```python
from build123d import *

# Parameters (mm, degrees)
SALIENTE_EXTRUIR3_DEPTH = 10
CROQUIS4_W              = 20
CROQUIS4_H              = 5
SALIENTE_EXTRUIR4_DEPTH = 10
CROQUIS5_W              = 5
CROQUIS5_H              = 5
SALIENTE_EXTRUIR5_DEPTH = 20
CORTAR_EXTRUIR1_DEPTH   = 2
CROQUIS8_W              = 20
CROQUIS8_H              = 5
CORTAR_EXTRUIR2_DEPTH   = 2
CROQUIS9_W              = 5
CROQUIS9_H              = 20
CORTAR_EXTRUIR3_DEPTH   = 2
CROQUIS10_W             = 20
CROQUIS10_H             = 5
CORTAR_EXTRUIR5_DEPTH   = 35
SALIENTE_EXTRUIR6_DEPTH = 5
CROQUIS12_W             = 26.103344273
CROQUIS12_H             = 18.453448341
CORTAR_EXTRUIR6_DEPTH   = 0.25


with BuildPart() as part:
    # Croquis1 → Saliente-Extruir3 (new body)
    with BuildSketch(Plane(origin=(0, 0, 0), x_dir=(1, 0, 0), z_dir=(0, 1, 0))):
        Polygon((-12.713671106, 38.358548308), (-10.713671106, 38.358548308), (-10.713671106, 39.358548308), (-15.713671106, 39.358548308), (-15.713671106, 19.358548308), (-10.713671106, 19.358548308), (-10.713671106, 20.358548308), (-12.713671106, 20.358548308), (-12.713671106, 21.358548308), (-10.718625385, 21.358548308), (-10.718625385, 37.358548308), (-12.713671106, 37.358548308), align=None)
    extrude(amount=SALIENTE_EXTRUIR3_DEPTH)



with BuildPart() as body_2:
    # Croquis4 → Saliente-Extruir4 (new body)
    with BuildSketch(Plane(origin=(-10.713671106, 0, 0), x_dir=(0, 0, -1), z_dir=(1, 0, 0))):
        with Locations((29.358548308, -2.5)):
            Rectangle(CROQUIS4_W, CROQUIS4_H)
    extrude(amount=SALIENTE_EXTRUIR4_DEPTH)


with BuildPart() as part_1:
    add(part.part)

    add(body_2.part)  # Saliente-Extruir5 merges body 2
    # Croquis5 → Saliente-Extruir5 (add)
    with BuildSketch(Plane.XY.offset(-19.358548308)):
        with Locations((-13.213671106, -2.5)):
            Rectangle(CROQUIS5_W, CROQUIS5_H)
    extrude(amount=-SALIENTE_EXTRUIR5_DEPTH)

    # Croquis7 → Cortar-Extruir1 (cut)
    with BuildSketch(Plane(origin=(0, 0, 0), x_dir=(1, 0, 0), z_dir=(0, 1, 0))):
        Polygon((-10.714909676, 37.358548308), (-0.713671106, 37.358548308), (-0.713671106, 38.358548308), (-10.713671106, 38.358548308), (-12.713671106, 38.358548308), (-12.713671106, 37.358548308), align=None)
        Polygon((-10.713671106, 20.358548308), (-0.713671106, 20.358548308), (-0.713671106, 21.358548308), (-10.714909676, 21.358548308), (-12.713671106, 21.358548308), (-12.713671106, 20.358548308), align=None)
    extrude(amount=-CORTAR_EXTRUIR1_DEPTH, mode=Mode.SUBTRACT)

    # Croquis8 → Cortar-Extruir2 (cut)
    with BuildSketch(Plane(origin=(-0.713671106, 0, 0), x_dir=(0, 0, -1), z_dir=(1, 0, 0))):
        with Locations((29.358548308, -2.5)):
            Rectangle(CROQUIS8_W, CROQUIS8_H)
    extrude(amount=-CORTAR_EXTRUIR2_DEPTH, mode=Mode.SUBTRACT)

    # Croquis9 → Cortar-Extruir3 (cut)
    with BuildSketch(Plane(origin=(0, 10, 0), x_dir=(1, 0, 0), z_dir=(0, 1, 0))):
        with Locations((-13.213671106, 29.358548308)):
            Rectangle(CROQUIS9_W, CROQUIS9_H)
    extrude(amount=-CORTAR_EXTRUIR3_DEPTH, mode=Mode.SUBTRACT)

    # Croquis10 → Cortar-Extruir5 (cut)
    with BuildSketch(Plane(origin=(-2.713671106, 0, 0), x_dir=(0, 0, -1), z_dir=(1, 0, 0))):
        with Locations((29.358548308, -2.5)):
            Rectangle(CROQUIS10_W, CROQUIS10_H)
    extrude(amount=-CORTAR_EXTRUIR5_DEPTH, mode=Mode.SUBTRACT)

    # Croquis11 → Saliente-Extruir6 (add)
    with BuildSketch(Plane.XZ):
        Polygon((-10.713671106, -20.358548308), (-10.713671106, -19.358548308), (-15.713671106, -19.358548308), (-15.713671106, -39.358548308), (-10.713671106, -39.358548308), (-10.713671106, -38.358548308), (-12.713671106, -38.358548308), (-12.713671106, -37.358548308), (-10.716767531, -37.358548308), (-10.717696458, -21.358548308), (-12.713671106, -21.358548308), (-12.713671106, -20.358548308), align=None)
    extrude(amount=SALIENTE_EXTRUIR6_DEPTH)

    # Croquis12 → Cortar-Extruir6 (cut)
    with BuildSketch(Plane(origin=(-10.713671106, 0, 0), x_dir=(0, 0, -1), z_dir=(1, 0, 0))):
        with Locations((28.040672231, 2.092138624)):
            Rectangle(CROQUIS12_W, CROQUIS12_H)
    extrude(amount=-CORTAR_EXTRUIR6_DEPTH, mode=Mode.SUBTRACT)


solid = part_1.part
```
Here's how the part is built. I have some questions about the finished solid (model axes, mm). A direction names the side the tool comes from. Give positions to 0.01 mm unless a question says otherwise; leave off trailing zeros. Order: outer loops, then holes, each group sorted by start corner. A loop starts at its lowest first (then second) coordinate and runs counter-clockwise, first axis right, second up. Notation, with made-up numbers: (-28, -35.75) - (-7, -35.75) arc R8 cw to (-7, -26.75) - close; hole circle Ø10 at (44, -4.5). An arc over 180 degrees is marked (long way). Answer as a JSON object with one key per item and string values. Group by question number.
Item 1: If we mould it in two halves opening along Z, with no side actions, what happens to faces 1 (the flat face through (-12, 2, -37.359)), 2 (the flat face through (-13, 2, -39.359)), 3 (the flat face through (-10.964, 2, -20)), 4 (the flat face through (-12, 2, -21.359))? For each: pulls with the +Z half, pulls with the -Z half, needs draft (parallel to the pull), parting line crosses it, or undercut.
Item 2: If we section it at A-A on y = 0.25: Please give me the cut outline in (x, z).
Item 3: Which directions (+Z, -Z, +X, -X, +Y, -Y) give clear straight access to the entire face, cutting with the end or side of a thin tool? Please do faces 5 (the flat face through (-12.714, 2, -21)), 6 (the flat face through (-13, -5, -29)).
Item 4: For P1, Ø0.5, axis at y = -0.5, z = -21, coming from the +X side, with a flat end and sliding along its axis, tell me the tip position at first contact or that it passes through.
Item 5: Please list where these lines run through material, in increasing order: probe 1 along Z at (x, y) = (-12.45, -1.5); probe 2 along X at (y, z) = (1, -37.5).
Item 6: If we section it at B-B on z = -37.75: Please give me the cut outline in (x, y).
Result set:
{
 "1": {"face 1": "undercut", "face 2": "pulls with the -Z half", "face 3": "needs draft", "face 4": "undercut"},
 "2": {"outline": "(-15.71, -39.36) - (-10.96, -39.36) - (-10.96, -38.36) - (-12.71, -38.36) - (-12.71, -37.36) - (-10.96, -37.36) - (-10.96, -21.36) - (-12.71, -21.36) - (-12.71, -20.36) - (-10.96, -20.36) - (-10.96, -19.36) - (-15.71, -19.36) - close"},
 "3": {"face 5": "+X, +Y, -Y", "face 6": "+Z, -Z, +X, -X, -Y"},
 "4": {"P1": "x = -12.71"},
 "5": {"probe 1": "-39.36 to -38.36, -37.36 to -21.36, -20.36 to -19.36", "probe 2": "-15.71 to -12.71"},
 "6": {"outline": "(-15.71, -5) - (-12.71, -5) - (-12.71, 8) - (-15.71, 8) - close"}
}
